from build123d import *

# Parameters (mm, degrees)
F0_W     = 100.0125
F0_H     = 127
F0_H_2   = 50.8
F0_W_2   = 11.1125
F1_DEPTH = 25.4


with BuildPart() as f1:
    # F0 (on Top) → F1 (new body)
    with BuildSketch(Plane.XY):
        with Locations((-305.59375, 215.9)):
            Rectangle(F0_W, F0_H)
        with Locations((-205.58125, 215.9)):
            Rectangle(F0_W, F0_H)
        with Locations((-305.59375, 88.9)):
            Rectangle(F0_W, F0_H)
        with Locations((-105.56875, 215.9)):
            Rectangle(F0_W, F0_H)
        with Locations((-305.59375, -38.1)):
            Rectangle(F0_W, F0_H)
        with Locations((-5.55625, 215.9)):
            Rectangle(F0_W, F0_H)
        with Locations((-305.59375, -165.1)):
            Rectangle(F0_W, F0_H)
        with Locations((94.45625, 215.9)):
            Rectangle(F0_W, F0_H)
        with Locations((-305.59375, -254)):
            Rectangle(F0_W, F0_H_2)
        with Locations((194.46875, 215.9)):
            Rectangle(F0_W, F0_H)
        with Locations((-205.58125, -254)):
            Rectangle(F0_W, F0_H_2)
        with Locations((294.48125, 215.9)):
            Rectangle(F0_W, F0_H)
        with Locations((-105.56875, -254)):
            Rectangle(F0_W, F0_H_2)
        with Locations((350.04375, 215.9)):
            Rectangle(F0_W_2, F0_H)
        with Locations((-5.55625, -254)):
            Rectangle(F0_W, F0_H_2)
        with Locations((350.04375, 88.9)):
            Rectangle(F0_W_2, F0_H)
        with Locations((94.45625, -254)):
            Rectangle(F0_W, F0_H_2)
        with Locations((350.04375, -38.1)):
            Rectangle(F0_W_2, F0_H)
        with Locations((194.46875, -254)):
            Rectangle(F0_W, F0_H_2)
        with Locations((350.04375, -165.1)):
            Rectangle(F0_W_2, F0_H)
        with Locations((294.48125, -254)):
            Rectangle(F0_W, F0_H_2)
        with Locations((350.04375, -254)):
            Rectangle(F0_W_2, F0_H_2)
    extrude(amount=F1_DEPTH)


solid = f1.part
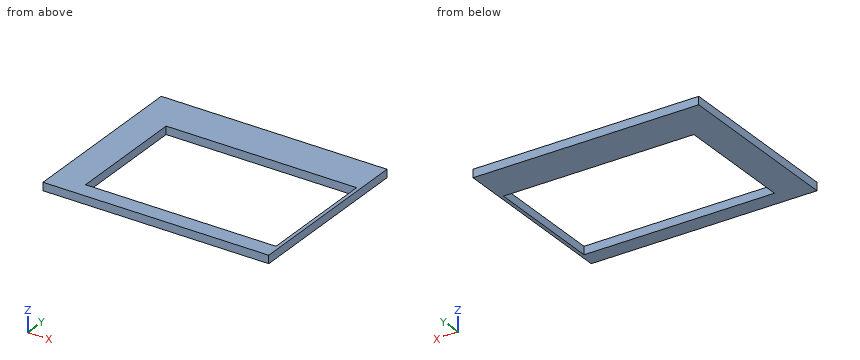
Geometry: final body of the model. Coordinates: model frame, mm. Give positions to 0.01 mm unless a question says otherwise; leave off trailing zeros. Write each loop counter-clockwise with the first axis right and the second up, starting at its lowest first coordinate (ties: lowest second). Pieces come first, ordered by that corner, then holes. Notation, with made-up numbers: M -2.5,-16.75 L 10.5,-16.75 A23 ccw 10.5,5.25 Z; hole C 54.5,25.25 d7. An arc over 180 degrees is marked long. Answer in a Markdown table with one row per item. Add a question column.
(1) Section A-A on y = 97. Return loops of the section in (x, z), and give its area (3 significant figures).
(2) Section C-C on x = 110.5. Return loops of the section in (y, z).
(3) Ray query, line 1 (Y direction, x = 217.5, z = 6.5); line 2 (X direction, y = 79.5, z = 2.25). Return the intervals inside material, ascending.
(4) Section B-B on z = 19. Return loops of the section in (x, y).
Result set:
| question | item | result |
|---|---|---|
| 1 | outline | M -355.6,0 L -255.59,0 L -255.59,25.4 L -355.6,25.4 Z; M 344.49,0 L 355.6,0 L 355.6,25.4 L 344.49,25.4 Z |
| 1 | area | 2,820 mm^2 |
| 2 | outline | M -279.4,0 L -228.6,0 L -228.6,25.4 L -279.4,25.4 Z; M 152.4,0 L 279.4,0 L 279.4,25.4 L 152.4,25.4 Z |
| 3 | line 1 | y = -279.4 to -228.6, 152.4 to 279.4 |
| 3 | line 2 | x = -355.6 to -255.59, 344.49 to 355.6 |
| 4 | outline | M -355.6,-279.4 L 355.6,-279.4 L 355.6,279.4 L -355.6,279.4 Z; hole M -255.59,-228.6 L 344.49,-228.6 L 344.49,152.4 L -255.59,152.4 Z |
